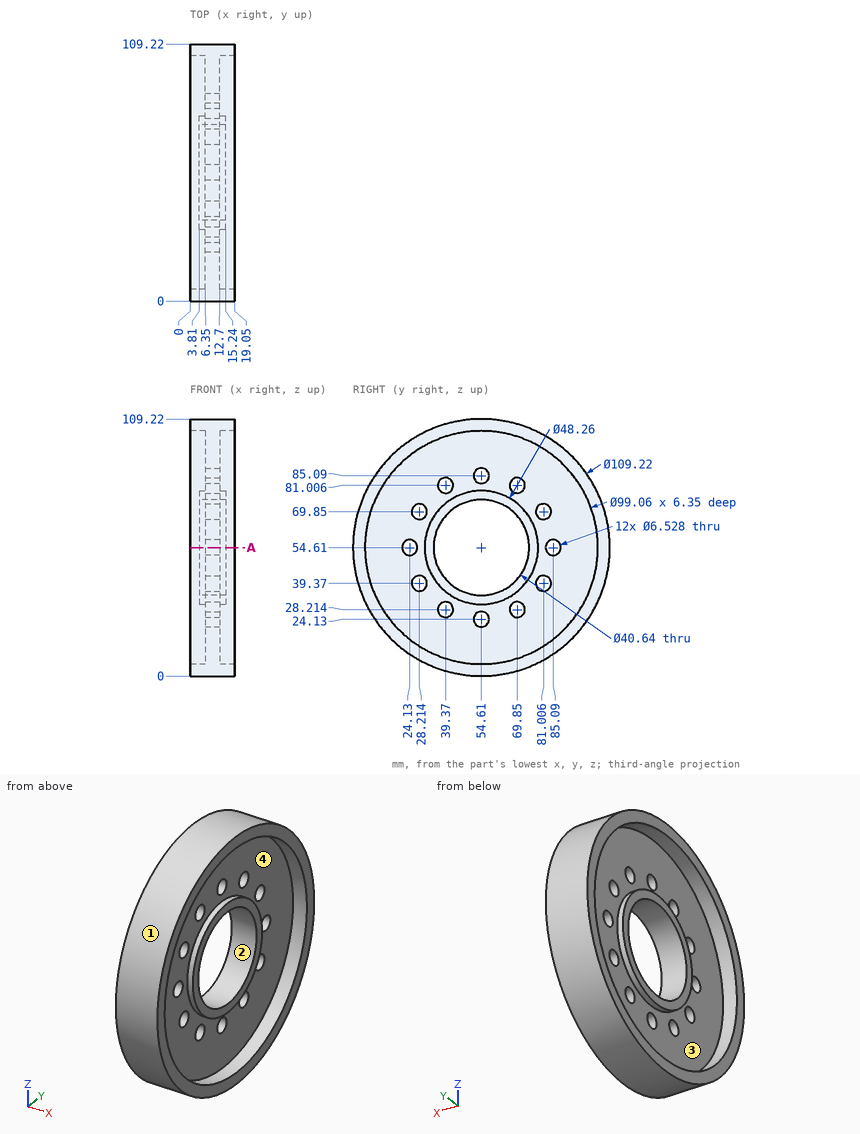
Print and shaded views of the part. All mm, measured from the part's lowest x, y and z. A direction names the side the tool comes from. Give positions to 0.01 mm unless a question says otherwise; leave off trailing zeros. Write each question's results on one line, items separated by ' | '.
Q1. Flat gauge pins, fed straight in: P1, Ø8.5, axis at y = 85.09, z = 54.61, coming from the -X side; P2, Ø10.5, axis at y = 54.61, z = 24.13, coming from the +X side; P3, Ø24, axis at y = 45, z = 52.5, coming from the +X side. Where does each tip first touch, or does it go through?
Geometry check:
P1: stops at x = 6.35 | P2: stops at x = 12.7 | P3: stops at x = 15.24
Q2. Mould opens along Y. For the marked faces 1 and 2 say: pulls with the +Y half, pulls with the -Y half, needs draft (parallel to the pull), parting line crosses it, or undercut.
Geometry check:
face 1: parting line crosses it | face 2: undercut
Q3. Probe probe 1 along Y at (x, z) = (12.75, 54.61); probe 2 along Y at (x, z) = (2, 54.61); probe 3 along X at (y, z) = (51, 11). List the from-to ranges inside material, lowest first.
Geometry check:
probe 1: y = 0 to 5.08, 30.48 to 34.29, 74.93 to 78.74, 104.14 to 109.22 | probe 2: y = 0 to 5.08, 104.14 to 109.22 | probe 3: x = 6.35 to 12.7
Q4. Band-saw the part on A-A on z = 54.61. Give the number of separate pieces and of enclosed holes in the cut face.
Geometry check:
separate pieces: 4 | enclosed holes: 0
Q5. Which spindle directions (+Z, -Z, +X, -X, +Y, -Y) get a long thin tool onto all of the face, cutting with end or side? Do the marked faces 3 and 4. Say none if no direction does.
Geometry check:
face 3: -X | face 4: +X
